from build123d import *

# Parameters (mm, degrees)
SKETCH1_R               = 4.6
SKETCH1_R_2             = 3.9
BOSS_EXTRUDE1_DEPTH     = 12
CUT_EXTRUDE1_DEPTH      = 6
SKETCH3_R               = 8
BOSS_EXTRUDE2_DEPTH     = 9.45
CUT_EXTRUDE2_DEPTH      = 3
SKETCH5_R               = 8
BOSS_EXTRUDE3_DEPTH     = 9.45
CUT_EXTRUDE3_DEPTH      = 3
CUT_EXTRUDE4_DEPTH      = 3
CUT_EXTRUDE4_DEPTH_BACK = 3
CUT_EXTRUDE5_DEPTH      = 3
CUT_EXTRUDE5_DEPTH_BACK = 3


with BuildPart() as part:
    # Sketch1 → Boss-Extrude1 (new body)
    with BuildSketch(Plane(origin=(0, 0, 0), x_dir=(1, 0, 0), z_dir=(0, 1, 0))):
        with BuildLine():
            Line((-17.5, -35), (17.5, -35))
            ThreePointArc((17.5, -35), (22.449747468, -32.949747468), (24.5, -28))
            Line((24.5, -28), (24.5, 28))
            ThreePointArc((24.5, 28), (22.449747468, 32.949747468), (17.5, 35))
            Line((17.5, 35), (-17.5, 35))
            ThreePointArc((-17.5, 35), (-22.449747468, 32.949747468), (-24.5, 28))
            Line((-24.5, 28), (-24.5, -28))
            ThreePointArc((-24.5, -28), (-22.449747468, -32.949747468), (-17.5, -35))
        make_face()
        with Locations((15.5, 28)):
            Circle(SKETCH1_R, mode=Mode.SUBTRACT)
        with Locations((15.5, -28)):
            Circle(SKETCH1_R, mode=Mode.SUBTRACT)
        with Locations((0, 28)):
            Circle(SKETCH1_R_2, mode=Mode.SUBTRACT)
        with Locations((0, -28)):
            Circle(SKETCH1_R_2, mode=Mode.SUBTRACT)
        with Locations((-15.5, 28)):
            Circle(SKETCH1_R, mode=Mode.SUBTRACT)
        with Locations((-15.5, -28)):
            Circle(SKETCH1_R, mode=Mode.SUBTRACT)
    extrude(amount=BOSS_EXTRUDE1_DEPTH)

    # Sketch2 → Cut-Extrude1 (cut)
    with BuildSketch(Plane(origin=(0, 0, 0), x_dir=(1, 0, 0), z_dir=(0, 1, 0))):
        with BuildLine():
            Line((-8.930372918, -22), (8.930372918, -22))
            ThreePointArc((8.930372918, -22), (9.298362954, -21.929829734), (9.614709072, -21.729166667))
            ThreePointArc((9.614709072, -21.729166667), (13.6405636, -19.603423539), (18.1875, -19.830707267))
            ThreePointArc((18.1875, -19.830707267), (19.08630197, -19.690882095), (19.5, -18.880789508))
            Line((19.5, -18.880789508), (19.5, 18.880789508))
            ThreePointArc((19.5, 18.880789508), (19.08630197, 19.690882095), (18.1875, 19.830707267))
            ThreePointArc((18.1875, 19.830707267), (13.6405636, 19.603423539), (9.614709072, 21.729166667))
            ThreePointArc((9.614709072, 21.729166667), (9.298362954, 21.929829734), (8.930372918, 22))
            Line((8.930372918, 22), (-8.930372918, 22))
            ThreePointArc((-8.930372918, 22), (-9.298362954, 21.929829734), (-9.614709072, 21.729166667))
            ThreePointArc((-9.614709072, 21.729166667), (-13.6405636, 19.603423539), (-18.1875, 19.830707267))
            ThreePointArc((-18.1875, 19.830707267), (-19.08630197, 19.690882095), (-19.5, 18.880789508))
            Line((-19.5, 18.880789508), (-19.5, -18.880789508))
            ThreePointArc((-19.5, -18.880789508), (-19.086301938, -19.690882118), (-18.187499925, -19.830707243))
            ThreePointArc((-18.187499925, -19.830707243), (-13.640563561, -19.603423547), (-9.614709072, -21.729166667))
            ThreePointArc((-9.614709072, -21.729166667), (-9.298362954, -21.929829734), (-8.930372918, -22))
        make_face()
    extrude(amount=CUT_EXTRUDE1_DEPTH, mode=Mode.SUBTRACT)

    # Sketch3 → Boss-Extrude2 (add)
    with BuildSketch(Plane.XY.offset(20)):
        with BuildLine():
            Line((-26.475934633, 49.095763671), (-24.5, 12))
            Line((-24.5, 12), (24.5, 12))
            Line((24.5, 12), (6.223487863, 56.463120719))
            ThreePointArc((6.223487863, 56.463120719), (-13.236528228, 66.584280413), (-26.475934633, 49.095763671))
        make_face()
        with Locations((-9.5, 50)):
            Circle(SKETCH3_R, mode=Mode.SUBTRACT)
    extrude(amount=-BOSS_EXTRUDE2_DEPTH)

    # Sketch4 → Cut-Extrude2 (cut)
    with BuildSketch(Plane.XY.offset(20)):
        with BuildLine():
            Line((-21.022370546, 40.713721035), (-19.543344466, 12.946809628))
            ThreePointArc((-19.543344466, 12.946809628), (-19.232804271, 12.274331215), (-18.544760076, 12))
            Line((-18.544760076, 12), (17.60184091, 12))
            ThreePointArc((17.60184091, 12), (18.432558544, 12.443305996), (18.526751961, 13.380183572))
            Line((18.526751961, 13.380183572), (4.891418921, 46.552238199))
            ThreePointArc((4.891418921, 46.552238199), (3.910016369, 47.170457707), (3.004614451, 46.445479297))
            ThreePointArc((3.004614451, 46.445479297), (-6.642654885, 37.317903214), (-19.272087144, 41.426417736))
            ThreePointArc((-19.272087144, 41.426417736), (-20.400909801, 41.693074328), (-21.022370546, 40.713721035))
        make_face()
    extrude(amount=-CUT_EXTRUDE2_DEPTH, mode=Mode.SUBTRACT)

    # Sketch5 → Boss-Extrude3 (add)
    with BuildSketch(Plane.XY.offset(-20)):
        with BuildLine():
            Line((-26.475934633, 49.095763671), (-24.5, 12))
            Line((-24.5, 12), (24.5, 12))
            Line((24.5, 12), (6.223487863, 56.463120719))
            ThreePointArc((6.223487863, 56.463120719), (-13.236528228, 66.584280413), (-26.475934633, 49.095763671))
        make_face()
        with Locations((-9.5, 50)):
            Circle(SKETCH5_R, mode=Mode.SUBTRACT)
    extrude(amount=BOSS_EXTRUDE3_DEPTH)

    # Sketch6 → Cut-Extrude3 (cut)
    with BuildSketch(Plane.XY.offset(-20)):
        with BuildLine():
            Line((-21.022370546, 40.713721035), (-19.543344466, 12.946809628))
            ThreePointArc((-19.543344466, 12.946809628), (-19.232804271, 12.274331215), (-18.544760076, 12))
            Line((-18.544760076, 12), (17.60184091, 12))
            ThreePointArc((17.60184091, 12), (18.432558544, 12.443305996), (18.526751961, 13.380183572))
            Line((18.526751961, 13.380183572), (4.891418921, 46.552238199))
            ThreePointArc((4.891418921, 46.552238199), (3.910016369, 47.170457707), (3.004614451, 46.445479297))
            ThreePointArc((3.004614451, 46.445479297), (-6.642654885, 37.317903214), (-19.272087144, 41.426417736))
            ThreePointArc((-19.272087144, 41.426417736), (-20.400909801, 41.693074328), (-21.022370546, 40.713721035))
        make_face()
    extrude(amount=CUT_EXTRUDE3_DEPTH, mode=Mode.SUBTRACT)

    # Sketch7 → Cut-Extrude4 (cut, two sides)
    with BuildSketch(Plane.XY.offset(20)) as cut_extrude4_sk:
        with BuildLine():
            Line((-7.35, 35.15), (-7.35, 50))
            Line((-7.35, 50), (-11.65, 50))
            Line((-11.65, 50), (-11.65, 35.15))
            ThreePointArc((-11.65, 35.15), (-9.5, 33), (-7.35, 35.15))
        make_face()
    extrude(amount=CUT_EXTRUDE4_DEPTH, mode=Mode.SUBTRACT)
    extrude(cut_extrude4_sk.sketch, amount=-CUT_EXTRUDE4_DEPTH_BACK, mode=Mode.SUBTRACT)

    # Sketch8 → Cut-Extrude5 (cut, two sides)
    with BuildSketch(Plane.XY.offset(-20)) as cut_extrude5_sk:
        with BuildLine():
            Line((-7.35, 35.15), (-7.35, 50))
            Line((-7.35, 50), (-11.65, 50))
            Line((-11.65, 50), (-11.65, 35.15))
            ThreePointArc((-11.65, 35.15), (-9.5, 33), (-7.35, 35.15))
        make_face()
    extrude(amount=CUT_EXTRUDE5_DEPTH, mode=Mode.SUBTRACT)
    extrude(cut_extrude5_sk.sketch, amount=-CUT_EXTRUDE5_DEPTH_BACK, mode=Mode.SUBTRACT)


solid = part.part
The model under review builds one solid part; all positions refer to its coordinate system, in mm. A direction names the side the tool comes from. Coordinates: 2 decimals unless noted, no trailing zeros. Write each loop counter-clockwise with the first axis right and the second up, starting at its lowest first coordinate (ties: lowest second). Pieces come first, ordered by that corner, then holes. Notation, with made-up numbers: (65, -5) -> (106, -5) arc R26 cw to (106, 25) -> close; hole circle Ø1 at (48.25, -32.5). An arc over 180 degrees is marked (long way). Answer in a Markdown table with one row per item.
1. Wall thickness on probe 1 along X at (y, z) = (6.75, 28); probe 2 along Z at (x, y) = (-10, 63); probe 3 along Z at (x, y) = (-15.5, 7): over which ranges is each line inside the solid? List them lowest first. Write a range as [from, to].
Answers below:
| item | result |
|---|---|
| probe 1 | x = [-24.5, -20.1], [-10.9, -3.9], [3.9, 10.9], [20.1, 24.5] |
| probe 2 | z = [-20, -10.55], [10.55, 20] |
| probe 3 | z = [-35, -32.6], [-23.4, 23.4], [32.6, 35] |
2. For faces 1 (the flat face through (0, 6, 0)), 2 (the flat face through (-20.293, 27.025, -18.521)), 3 (the cylindrical face through (3.93, 47.17, 18.52)), 4 (the flat face through (21, 0, 0)), list the 3-axis set-ups (+Z, -Z, +X, -X, +Y, -Y) from which the entire face can be reached by the end or side of a thin tool; tool diameter is ignored.
Answers below:
| item | result |
|---|---|
| face 1 | -Y |
| face 2 | -Z |
| face 3 | +Z |
| face 4 | +Z, -Z, +X, -X, -Y |
3. Clearance check with flat-ended pins moving along their axes: pin 1 Ø10.5 at (x, y) = (5, 27.5) entering from -Z; pin 2 Ø2.5 at (y, z) = (40.5, -18) entering from -X; pin 3 Ø14.5 at (x, z) = (2, -29) entering from +Y; pin 4 Ø8 at (x, y) = (17.5, 43.5) entering from +Z. State where each tip first meets the part, or that it passes through.
Answers below:
| item | result |
|---|---|
| pin 1 | stops at z = -17 |
| pin 2 | stops at x = -26.08 |
| pin 3 | stops at y = 12 |
| pin 4 | passes through |
4. We need section C-C, the plane x = 13.5. State the section outline as (y, z) points.
Answers below:
| item | result |
|---|---|
| outline | (0, -35) -> (12, -35) -> (12, -32.14) -> (0, -32.14) -> close; (0, -23.86) -> (12, -23.86) -> (12, -17) -> (25.61, -17) -> (25.61, -20) -> (38.76, -20) -> (38.76, -10.55) -> (12, -10.55) -> (12, 10.55) -> (38.76, 10.55) -> (38.76, 20) -> (25.61, 20) -> (25.61, 17) -> (12, 17) -> (12, 23.86) -> (0, 23.86) -> (0, 19.64) -> (6, 19.64) -> (6, -19.64) -> (0, -19.64) -> close; (0, 32.14) -> (12, 32.14) -> (12, 35) -> (0, 35) -> close |
5. Draft analysis for pull direction X (two halves, no side actions). For faces 5 (the flat face through (-7, 34, -10.55)), 6 (the flat face through (-24.5, 6, 0)), 7 (the flat face through (-19.5, 3, 0)), state which applies: +X half, -X half, draft (parallel to the pull), parting line (faces both ways), or undercut.
Answers below:
| item | result |
|---|---|
| face 5 | draft |
| face 6 | -X half |
| face 7 | undercut |
6. We need section D-D, the plane y = 7.5. State the section outline as (x, z) points.
Answers below:
| item | result |
|---|---|
| outline | (-24.5, -28) arc R7 ccw to (-17.5, -35) -> (17.5, -35) arc R7 ccw to (24.5, -28) -> (24.5, 28) arc R7 ccw to (17.5, 35) -> (-17.5, 35) arc R7 ccw to (-24.5, 28) -> close; hole circle Ø9.2 at (-15.5, -28); hole circle Ø9.2 at (-15.5, 28); hole circle Ø7.8 at (0, -28); hole circle Ø7.8 at (0, 28); hole circle Ø9.2 at (15.5, -28); hole circle Ø9.2 at (15.5, 28) |
7. We need section A-A, the plane z = 14.5. State the section outline as (x, y) points.
Answers below:
| item | result |
|---|---|
| outline | (-26.48, 49.1) -> (-24.5, 12) -> (-24.5, 0) -> (-19.5, 0) -> (-19.5, 6) -> (19.5, 6) -> (19.5, 0) -> (24.5, 0) -> (24.5, 12) -> (6.22, 56.46) arc R17 ccw to start; hole circle Ø16 at (-9.5, 50) |
